from build123d import *

# Parameters (mm, degrees)
SKETCH1_W           = 19.304
SKETCH1_H           = 70.104
BOSS_EXTRUDE1_DEPTH = 609.6
SKETCH2_W           = 3.175
SKETCH2_H           = 38.1
CUT_EXTRUDE1_DEPTH  = 38.1
LPATTERN1_COUNT     = 17
LPATTERN1_PITCH     = 27.74188
FILLET1_R           = 3.81
SKETCH4_R           = 2.625
CUT_EXTRUDE2_DEPTH  = 6.35
LPATTERN2_COUNT     = 2
LPATTERN2_PITCH     = 507.1999


with BuildPart() as part:
    # Sketch1 → Boss-Extrude1 (new body)
    with BuildSketch(Plane(origin=(0, 0, 0), x_dir=(0, 0, -1), z_dir=(1, 0, 0))):
        with BuildLine():
            Line((3.048, 0), (22.352, 0))
            ThreePointArc((22.352, 0), (24.507261469, 0.892738531), (25.4, 3.048))
            Line((25.4, 3.048), (25.4, 73.152))
            ThreePointArc((25.4, 73.152), (24.507261469, 75.307261469), (22.352, 76.2))
            Line((22.352, 76.2), (3.048, 76.2))
            ThreePointArc((3.048, 76.2), (0.892738531, 75.307261469), (0, 73.152))
            Line((0, 73.152), (0, 3.048))
            ThreePointArc((0, 3.048), (0.892738531, 0.892738531), (3.048, 0))
        make_face()
        with Locations((12.7, 38.1)):
            Rectangle(SKETCH1_W, SKETCH1_H, mode=Mode.SUBTRACT)
    extrude(amount=BOSS_EXTRUDE1_DEPTH)

    # Sketch2 → Cut-Extrude1 (cut)
    with BuildSketch(Plane(origin=(0, 76.2, 0), x_dir=(1, 0, 0), z_dir=(0, 1, 0))):
        with Locations((82.8675, 22.098)):
            Rectangle(SKETCH2_W, SKETCH2_H)
    cut_extrude1 = extrude(amount=-CUT_EXTRUDE1_DEPTH, mode=Mode.SUBTRACT)

    # LPattern1: Cut-Extrude1 ×17
    with Locations(*[(i * LPATTERN1_PITCH, 0, 0) for i in range(1, LPATTERN1_COUNT)]):
        add(cut_extrude1, mode=Mode.SUBTRACT)

    # Fillet1
    # the kernel refuses this fillet: 3.81 mm, written as the material it takes off along each edge
    with BuildSketch(Plane(origin=(609.6, 0, 6.477), x_dir=(0, 1, 0), z_dir=(0, 0, -1))) as fillet1_piece_1:
        with BuildLine():
            CenterArc((FILLET1_R, -FILLET1_R), FILLET1_R, 90, 90)
            Line((0, -FILLET1_R), (0, 0))
            Line((0, 0), (FILLET1_R, 0))
        make_face()
    extrude(amount=38.354, mode=Mode.SUBTRACT)
    with BuildSketch(Plane(origin=(0, 0, 6.477), x_dir=(0, 1, 0), z_dir=(0, 0, -1))) as fillet1_piece_2:
        with BuildLine():
            CenterArc((FILLET1_R, FILLET1_R), FILLET1_R, 180, 90)
            Line((0, FILLET1_R), (0, 0))
            Line((0, 0), (FILLET1_R, 0))
        make_face()
    extrude(amount=38.354, mode=Mode.SUBTRACT)

    # Sketch4 → Cut-Extrude2 (cut)
    with BuildSketch(Plane(origin=(0, 0, -25.4), x_dir=(-1, 0, 0), z_dir=(0, 0, -1))):
        with Locations((-578.4038, 62.073165047)):
            Circle(SKETCH4_R)
        with Locations((-538.4038, 62.073165047)):
            Circle(SKETCH4_R)
        with Locations((-540.0688, 15.723165047)):
            Circle(SKETCH4_R)
        with Locations((-576.3188, 15.723165047)):
            Circle(SKETCH4_R)
    cut_extrude2 = extrude(amount=-CUT_EXTRUDE2_DEPTH, mode=Mode.SUBTRACT)

    # LPattern2: Cut-Extrude2 ×2
    with Locations(*[(-i * LPATTERN2_PITCH, 0, 0) for i in range(1, LPATTERN2_COUNT)]):
        add(cut_extrude2, mode=Mode.SUBTRACT)


solid = part.part
Here's how the part is built. I have some questions about the finished solid (model axes, mm). A direction names the side the tool comes from. Round coordinates to 2 decimals unless told otherwise and drop trailing zeros. Loops run counter-clockwise (first coordinate to the right, second up) from the corner with the lowest first, then second, coordinate; pieces in that order, holes last. Notation, with made-up numbers: M -23.75,69 L -19.75,69 A11 ccw -19.75,85 Z; hole C 64,54 d10. An arc over 180 degrees is marked long. Write each question's results on one line, items separated by ' | '. Start each with the question number.
(1) On a 3-axis mill with a long thin cutter (end or side, diameter ignored), from which of +Z, -Z, +X, -X, +Y, -Y can I reach the whole of each face in a straight line? I mean faces 1 (the flat face through (429, 76.2, -13)), 2 (the flat face through (358.699, 63, -23)), 3 (the flat face through (235, 73.152, -13)). Say none if no direction works.
(2) Will these pins go through, and if not, where does the flat tip stop? P1, Ø2.5, axis at x = 194.5, z = -23.5, coming from the +Y side; P2, Ø0.9, axis at x = 444, z = -23.5, coming from the +Y side; P3, Ø6, axis at x = 388.5, y = 40, coming from the -Z side; P4, Ø3, axis at x = 538.4, y = 62.07, coming from the -Z side.
(3) I want a section at A-A (y = 27.5). Please give me the cut outline in (x, z).
(4) Thinking about a two-plate mould opening in X: for faces 4 (the flat face through (609.6, 43, -23)), 5 (the flat face through (235, 76.2, -13)), 6 (the flat face through (445.099, 63, -23)), 7 (the flat face through (195.423, 63, -23)), which applies, pulls with the +X half, pulls with the -X half, needs draft (parallel to the pull), parting line crosses it, or undercut?
(5) If I drill on probe 1 along Z at (x, y) = (213, 25.5); probe 2 along Y at (x, z) = (270.5, -14.25); probe 3 along Y at (x, z) = (165, -22), over which ranges is the centre line in solid material (lowest first)? Write a range as from..to.
(6) I want a section at C-C (z = -8.75). State how many separate pieces and enclosed holes the cut face has, then the cut area to 3 significant figures.
(7) I want a section at B-B (x = 264.5). Please give me the cut outline in (y, z).
Solved:
1) face 1: +Z, -Z, +X, -X, +Y | face 2: -Z, +Y | face 3: +X, -X
2) P1: stops at y = 76.18 | P2: stops at y = 38.1 | P3: stops at z = -25.4 | P4: stops at z = -3.05
3) outline: M 0,-25.4 L 609.6,-25.4 L 609.6,-22.35 L 0,-22.35 Z; M 0,-3.05 L 609.6,-3.05 L 609.6,0 L 0,0 Z
4) face 4: pulls with the +X half | face 5: needs draft | face 6: undercut | face 7: undercut
5) probe 1: z = -25.4..-22.35, -3.05..0 | probe 2: y = 0..3.05, 73.15..76.2 | probe 3: y = 0..3.05
6) separate pieces: 19 | enclosed holes: 0 | area: 3,550 mm²
7) outline: M 0,-22.35 A3.05 ccw 3.05,-25.4 L 73.15,-25.4 A3.05 ccw 76.2,-22.35 L 76.2,-3.05 A3.05 ccw 73.15,0 L 3.05,0 A3.05 ccw 0,-3.05 Z; hole M 3.05,-22.35 L 73.15,-22.35 L 73.15,-3.05 L 3.05,-3.05 Z
